Check sheet for the drawn part. Datum: minimum x, y, z corner. Units: mm. Give positions to 0.01 mm unless a question says otherwise; leave off trailing zeros. Loops run counter-clockwise (first coordinate to the right, second up) from the corner with the lowest first, then second, coordinate; pieces in that order, holes last. Notation, with made-up numbers: (-4, -36.75) - (11, -36.75) arc R30 cw to (11, -13.75) - close; hole circle Ø5 at (9.25, 75.25). An arc over 180 degrees is marked (long way). Use a Markdown table: item, result. Add a question column.
1. Depth check by flat-ended pin: P1, Ø2, axis at x = 61, y = 20.5, coming from the -Z side; P2, Ø5.5, axis at x = 25.4, y = 76.2, coming from the +Z side (3 decimals). Enter the tip coordinate at first touch or a pass-through.
2. Cross-section at B-B on y = 76.2. Enter the section's corners in (x, z) (3 decimals), and give its area (3 significant figures).
3. Material ranges on L1, parallel to Y at x = 25.4, z = 5 (3 decimals); L2, parallel to Y at x = 76.2, z = 10.25; L3, parallel to X at y = 76, z = 17, recorded low to high.
4. Draft check along X on the marked faces 1, 2, 3 and 4. Enter one of: pulls with the +X half, pulls with the -X half, needs draft (parallel to the pull), parting line crosses it, or undercut.
5. Cross-section at A-A on x = 76.2. Enter the section's corners in (y, z).
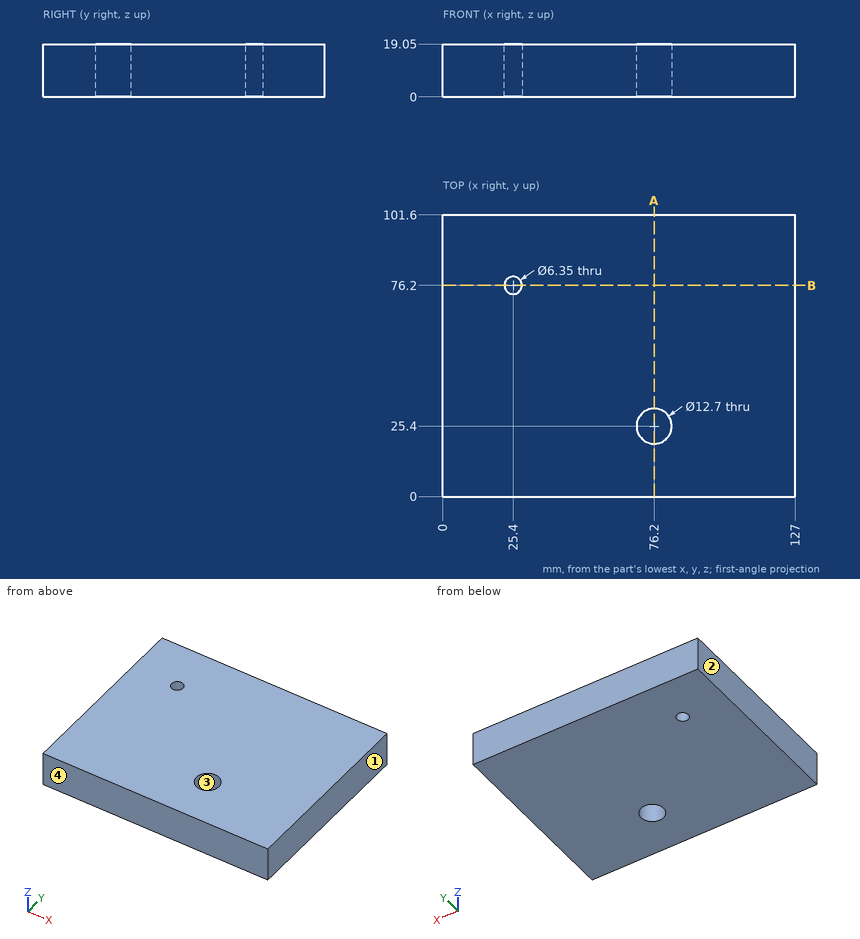
Values found:
| question | item | result |
|---|---|---|
| 1 | P1 | stops at z = 0 |
| 1 | P2 | passes through |
| 2 | outline | (0, 0) - (22.225, 0) - (22.225, 19.05) - (0, 19.05) - close; (28.575, 0) - (127, 0) - (127, 19.05) - (28.575, 19.05) - close |
| 2 | area | 2,300 mm2 |
| 3 | L1 | y = 0 to 73.025, 79.375 to 101.6 |
| 3 | L2 | y = 0 to 19.05, 31.75 to 101.6 |
| 3 | L3 | x = 0 to 22.23, 28.57 to 127 |
| 4 | face 1 | pulls with the +X half |
| 4 | face 2 | pulls with the -X half |
| 4 | face 3 | undercut |
| 4 | face 4 | needs draft |
| 5 | outline | (0, 0) - (19.05, 0) - (19.05, 19.05) - (0, 19.05) - close; (31.75, 0) - (101.6, 0) - (101.6, 19.05) - (31.75, 19.05) - close |
